Autodesk Inventor part; units mm, degrees
ref_plane "YZ Plane" through (0, 0, 0) normal (1, 0, 0) x (0, 1, 0)
ref_plane "XZ Plane" through (0, 0, 0) normal (0, 1, 0) x (-1, 0, 0)
ref_plane "XY Plane" through (0, 0, 0) normal (0, 0, 1) x (1, 0, 0)
sketch "Sketch1" plane through (0, 0, 0) normal (0, 1, 0) x (-1, 0, 0)
  line L0 (15, 0) -> (15, -15)
  line L1 (15, -15) -> (0, -15)
  line L2 (0, -15) -> (0, -12)
  line L3 (0, -12) -> (12, -12)
  line L4 (12, -12) -> (12, 0)
  line L5 (12, 0) -> (15, 0)
  point P0 (0, 0)
  dimension "d0" = 15
  dimension "d1" = 15
  dimension "d10" = 3
  dimension "d11" = 12
  dimension "d12" = 12
extrude "Extrusion1" add sketch "Sketch1" along normal blind 86
sketch "Sketch4" plane through (-12, 0, 0) normal (1, 0, 0) x (0, 0, -1)
  line L0 (0, 0) -> (0, 86)
  line L1 (12, 0) -> (12, 86)
  line L2 (0, 86) -> (12, 86)
  line L3 (12, 86) -> (12, 83)
  line L4 (12, 83) -> (0, 83)
  line L5 (0, 83) -> (0, 86)
  dimension "d13" = 3
extrude "Extrusion3" add sketch "Sketch4" along normal blind 3.1
sketch "Sketch6" plane through (-12, 0, -12) normal (0, 0, 1) x (1, 0, 0)
  line L0 (3.1, 86) -> (12, 86)
  line L1 (12, 86) -> (3.1, 86)
  line L2 (3.1, 86) -> (3.1, 83)
  line L3 (3.1, 83) -> (12, 83)
  line L4 (12, 83) -> (12, 86)
  point P0 (12, 0)
extrude "Extrusion4" add sketch "Sketch6" along normal blind 12
fillet "Fillet3" radius 2 7 edges at (-7.5, 86, -15) (-15, 86, -7.5) (-15, 43, -15) (0, 43, -15) (-7.5, 86, 0) (0, 86, -7.5) (-15, 43, 0)
sketch "Sketch11" plane through (0, 86, 0) normal (0, 1, 0) x (1, 0, 0)
  arc A0 (-15, 2) -> (-13, 0) centre (-13, 2) ccw
  line L0 (-13, 0) -> (-10, 0)
  line L1 (-15, 9) -> (-15, 0)
  line L2 (-15, 0) -> (-13, 0)
  line L3 (-9, 9) -> (-9, 0)
  line L4 (-9, 0) -> (-15, 0)
  line L5 (-9, 9) -> (-15, 9)
  point P0 (0, 0)
  point P1 (-13, 0)
extrude "Extrusion7" cut sketch "Sketch11" against normal blind 6.1
sketch "Sketch12" plane through (-12, 0, 0) normal (1, 0, 0) x (0, 0, -1)
  line L0 (0, 33) -> (9, 33) construction
  line L1 (0, 38.9) -> (0, 36)
  line L2 (9, 36) -> (9, 38.9)
  line L3 (0, 36) -> (0, 38.9)
  line L4 (9, 36) -> (9, 35.9)
  line L5 (9, 38.9) -> (0, 38.9)
  line L6 (9, 38.9) -> (9, 35.8)
  line L7 (9, 35.8) -> (0, 35.8)
  line L8 (0, 0) -> (0, 79.9)
  line L9 (0, 35.8) -> (0, 38.9)
  dimension "d49" = 3.1
  dimension "d50" = 9
extrude "Extrusion8" cut sketch "Sketch12" against normal through all
properties part number "DoosjeHoeken" material "ABS Plastic"
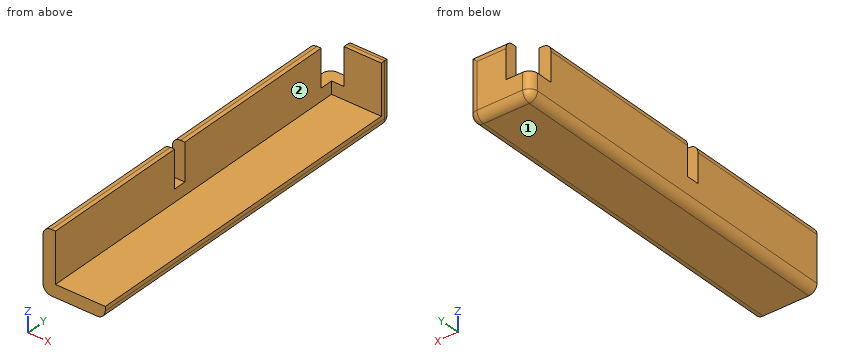
Verification items for the finished model (mm, model axes). Face numbers are marked on the shaded views. A direction names the side the tool comes from. Coordinates: 2 decimals unless noted, no trailing zeros. Write each loop counter-clockwise with the first axis right and the second up, starting at its lowest first coordinate (ties: lowest second). Pieces come first, ordered by that corner, then holes. Notation, with made-up numbers: (4, 36.25) - (46, 36.25) arc R4 ccw to (46, 40.25) - close; hole circle Ø9 at (33, 8). An arc over 180 degrees is marked (long way). One line per question, with ' | ' between items. Start each with the question number.
1. Material ranges on line 1 along Z through (x, y) = (-2.5, 15); line 2 along Y through (x, z) = (-5.25, -7.25), recorded low to high.
2. Section check B-B (y = 61). Enter the section's corners in (x, z), plus the area to 3 significant figures.
3. Section check A-A (z = -2.75). Enter the section's corners in (x, y).
4. Section check C-C (z = -11.25). Enter the section's corners in (x, y), plus the area to 3 significant figures.
5. Gauge pin test, flat ends, axial feed: P1, Ø5, axis at x = -4.5, z = -5.5, coming from the -Y side; P2, Ø6.5, axis at x = -13.5, y = 83.5, coming from the +Z side; P3, Ø0.9, axis at y = 85, z = -3, coming from the -X side. Record the tip position at first contact, or that the pin passes through.
6. Access from +Z, -Z, +X, -X, +Y, -Y to the whole of each face (thin tool, end or side, straight path). Record for the marked faces 1 and 2.
7. Section check D-D (x = -6.75). Enter the section's corners in (y, z), plus the area to 3 significant figures.
Computed values:
1) line 1: -15 to -12 | line 2: 83 to 86
2) outline: (-15, -13) arc R2 ccw to (-13, -15) - (-2, -15) arc R2 ccw to (0, -13) - (0, -12) - (-12, -12) - (-12, 0) - (-13, 0) arc R2 ccw to (-15, -2) - close | area: 78.4 mm²
3) outline: (-15, 0) - (-12, 0) - (-12, 35.8) - (-15, 35.8) - close; (-15, 38.9) - (-12, 38.9) - (-12, 79.9) - (-15, 79.9) - close; (-9, 83) - (0, 83) - (0, 84) arc R2 ccw to (-2, 86) - (-9, 86) - close
4) outline: (-15, 0) - (-12, 0) - (-12, 83) - (0, 83) - (0, 84) arc R2 ccw to (-2, 86) - (-13, 86) arc R2 ccw to (-15, 84) - close | area: 292 mm²
5) P1: y = 83 | P2: z = -9 | P3: x = -9
6) face 1: -Z, +X, -X, +Y, -Y | face 2: +Z, +X, -Y
7) outline: (0, -15) - (84, -15) arc R2 ccw to (86, -13) - (86, -2) arc R2 ccw to (84, 0) - (83, 0) - (83, -12) - (0, -12) - close | area: 292 mm²
